```python
from build123d import *

# Parameters (mm, degrees)
BOSS_EXTRUDE1_DEPTH = 2.5
SKETCH2_R           = 3
CUT_EXTRUDE1_DEPTH  = 2.5


with BuildPart() as part:
    # Sketch1 → Boss-Extrude1 (new body)
    with BuildSketch(Plane(origin=(0, 0, 0), x_dir=(1, 0, 0), z_dir=(0, 1, 0))):
        with BuildLine():
            Line((-3.769046254, -18.94827508), (-419.444192335, -2108.688352867))
            ThreePointArc((-419.444192335, -2108.688352867), (0, -2150), (419.444192335, -2108.688352867))
            Line((419.444192335, -2108.688352867), (3.769046254, -18.94827508))
            ThreePointArc((3.769046254, -18.94827508), (0, -16.086966015), (-3.769046254, -18.94827508))
        make_face()
    extrude(amount=BOSS_EXTRUDE1_DEPTH)

    # Sketch2 → Cut-Extrude1 (cut)
    with BuildSketch(Plane(origin=(0, 2.5, 0), x_dir=(1, 0, 0), z_dir=(0, 1, 0))):
        with Locations((-393.622932114, -2045.511913266)):
            Circle(SKETCH2_R)
        with Locations((-357.141041897, -1862.105065831)):
            Circle(SKETCH2_R)
        with Locations((-320.65915168, -1678.698218395)):
            Circle(SKETCH2_R)
        with Locations((-284.177261463, -1495.29137096)):
            Circle(SKETCH2_R)
        with Locations((-247.695371246, -1311.884523525)):
            Circle(SKETCH2_R)
        with Locations((-211.213481029, -1128.477676089)):
            Circle(SKETCH2_R)
        with Locations((-174.731590812, -945.070828654)):
            Circle(SKETCH2_R)
        with Locations((-138.249700595, -761.663981218)):
            Circle(SKETCH2_R)
        with Locations((-101.767810378, -578.257133783)):
            Circle(SKETCH2_R)
        with Locations((-65.285920161, -394.850286348)):
            Circle(SKETCH2_R)
        with Locations((65.285920161, -394.850286348)):
            Circle(SKETCH2_R)
        with Locations((101.767810378, -578.257133783)):
            Circle(SKETCH2_R)
        with Locations((138.249700595, -761.663981218)):
            Circle(SKETCH2_R)
        with Locations((174.731590812, -945.070828654)):
            Circle(SKETCH2_R)
        with Locations((211.213481029, -1128.477676089)):
            Circle(SKETCH2_R)
        with Locations((247.695371246, -1311.884523525)):
            Circle(SKETCH2_R)
        with Locations((284.177261463, -1495.29137096)):
            Circle(SKETCH2_R)
        with Locations((320.65915168, -1678.698218395)):
            Circle(SKETCH2_R)
        with Locations((357.141041897, -1862.105065831)):
            Circle(SKETCH2_R)
        with Locations((393.622932114, -2045.511913266)):
            Circle(SKETCH2_R)
        with Locations((0, -80)):
            Circle(SKETCH2_R)
    extrude(amount=-CUT_EXTRUDE1_DEPTH, mode=Mode.SUBTRACT)


solid = part.part
```
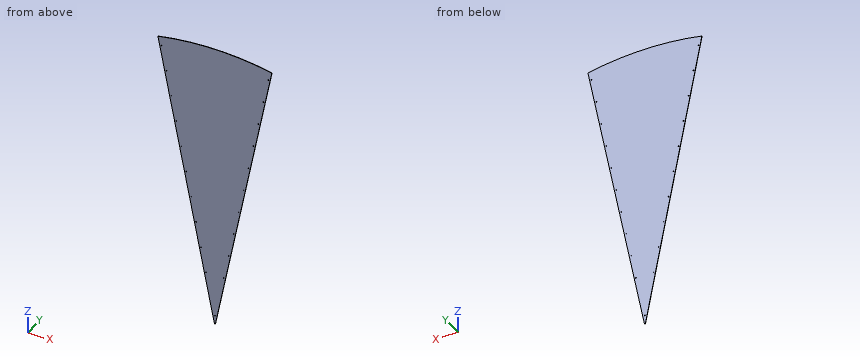
Input: part model. Units: mm. Frame: model coordinates. Round coordinates to 2 decimals unless told otherwise and drop trailing zeros. Loops run counter-clockwise (first coordinate to the right, second up) from the corner with the lowest first, then second, coordinate; pieces in that order, holes last. Notation, with made-up numbers: (60, -27.75) -> (100, -27.75) arc R5 cw to (100, -23.75) -> close; hole circle Ø11 at (4.25, 22). An arc over 180 degrees is marked (long way). Write each question's results on one line, items separated by ' | '.
1. Section C-C (z = 1169.5). Return loops of the section in (x, y).
Geometry results:
outline: (-232.63, 0) -> (232.63, 0) -> (232.63, 2.5) -> (-232.63, 2.5) -> close
2. First-contact query: P1, Ø5.5, axis at x = -138.25, z = 761.66, coming from the +Y side. Flat tip, straight axial feed; report the tip coordinate or a pass-through.
Geometry results:
P1: through
3. Section A-A (y = 0.4). State how many separate pieces and enclosed holes the cut face has, and give its area (3 significant figures).
Geometry results:
separate pieces: 1 | enclosed holes: 21 | area: 907,000 mm2
4. Section B-B (z = 1885.5). Return loops of the section in (x, y).
Geometry results:
outline: (-375.05, 0) -> (375.05, 0) -> (375.05, 2.5) -> (-375.05, 2.5) -> close
5. Ray query, line 1 (X direction, y = 0.4, z = 1677); line 2 (X direction, y = 0.55, z = 761); line 3 (X direction, y = 1.95, z = 862.5). Return the intervals inside material, ascending. Write a range as from..to.
Geometry results:
line 1: -333.58..-323.13, -318.19..318.19, 323.13..333.58 | line 2: -151.37..-141.18, -135.32..135.32, 141.18..151.37 | line 3: -171.56..171.56
